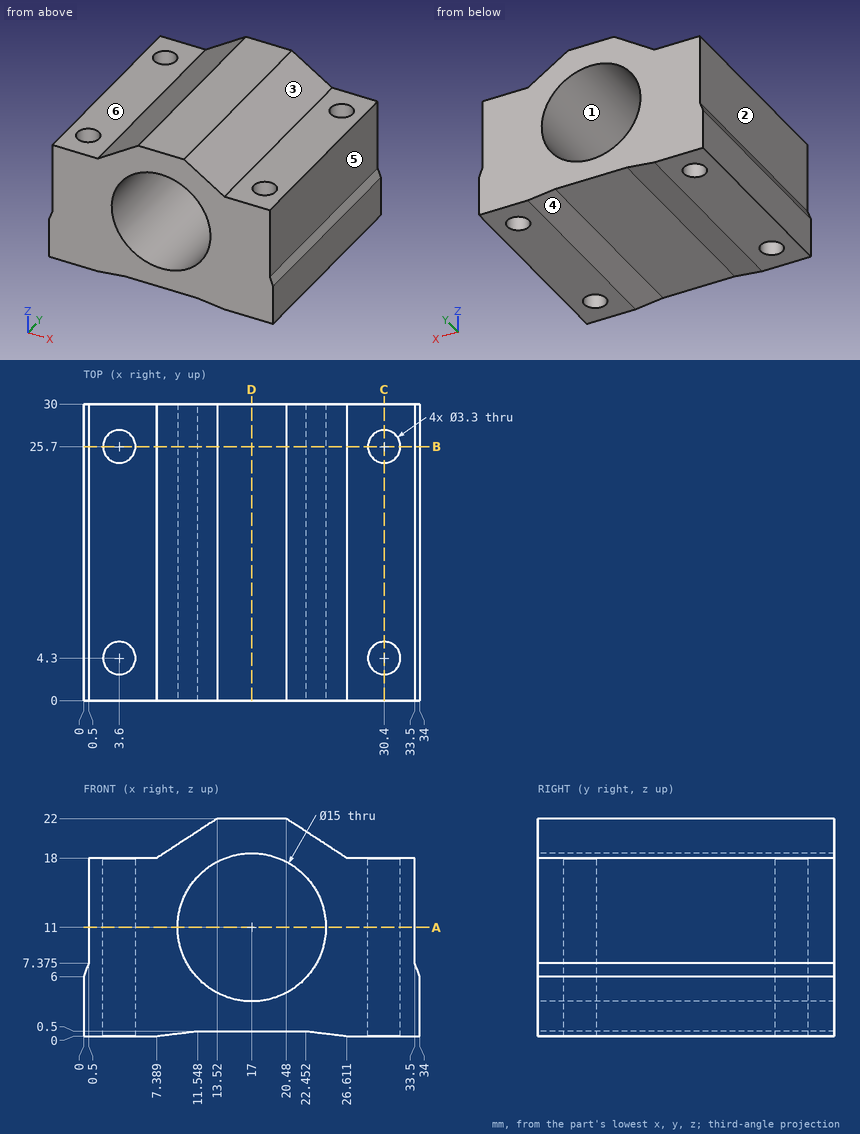
Study the drawing (mm; zero at the part's minimum x, y, z) and answer. A direction names the side the tool comes from. Coordinates: 2 decimals unless noted, no trailing zeros. Write each loop counter-clockwise with the first axis right and the second up, starting at its lowest first coordinate (ties: lowest second). Pieces come first, ordered by that corner, then holes. Notation, with made-up numbers: M 58.5,40.25 L 72.5,40.25 A23 ccw 72.5,59.25 Z; hole C 42.5,23 d1. An arc over 180 degrees is marked long. Write each question's results on one line, items separated by ' | '.
Item 1: Given P1, Ø8, axis at x = 8.5, y = 27, coming from the -Z side; P2, Ø2.5, axis at x = 3.6, y = 4.3, coming from the +Z side; P3, Ø5.5, axis at x = 19, y = 9.5, coming from the -Z side; P4, Ø8, axis at x = 7, y = 20, coming from the +Z side (1 decimal), each flat-ended and moving along its own axis, determine where each tip first touches the part or whether it passes through.
Answer below:
P1: z = 0 | P2: through | P3: z = 0.5 | P4: z = 20.4
Item 2: For a pull along X with two mould halves and no side action, classify the marked faces 1, 2 and 3 as released by +X, released by -X, zero draft, split by the parting line, or undercut.
Answer below:
face 1: undercut | face 2: released by -X | face 3: released by +X
Item 3: The part is cut by section D-D on x = 17. Determine the outline of the cut face in (y, z).
Answer below:
outline: M 0,0.5 L 30,0.5 L 30,3.5 L 0,3.5 Z; M 0,18.5 L 30,18.5 L 30,22 L 0,22 Z
Item 4: The part is cut by section A-A on z = 11. Determine the outline of the cut face in (x, y).
Answer below:
outline: M 0.5,0 L 9.5,0 L 9.5,30 L 0.5,30 Z; M 24.5,0 L 33.5,0 L 33.5,30 L 24.5,30 Z; hole C 3.6,4.3 d3.3; hole C 3.6,25.7 d3.3; hole C 30.4,4.3 d3.3; hole C 30.4,25.7 d3.3
Item 5: Which of the six approach directions +Z, -Z, +X, -X, +Y, -Y give full straight-line access (tool end or side, diameter ignored) to the marked faces 4, 5 and 6?
Answer below:
face 4: -Z, +Y, -Y | face 5: +Z, +X, +Y, -Y | face 6: +Z, -X, +Y, -Y
Item 6: The part is cut by section C-C on x = 30.4. Determine the outline of the cut face in (y, z), and give its area (3 significant figures).
Answer below:
outline: M 0,0 L 2.65,0 L 2.65,18 L 0,18 Z; M 5.95,0 L 24.05,0 L 24.05,18 L 5.95,18 Z; M 27.35,0 L 30,0 L 30,18 L 27.35,18 Z | area: 421 mm2
Item 7: Consider probe 1 along Y at (x, z) = (3.6, 4); probe 2 along Y at (x, z) = (3, 11.25); probe 3 along X at (y, z) = (25, 3.25) (1 decimal). Determine where each line is inside the solid, lowest interval first. Write a range as [from, to].
Answer below:
probe 1: [0, 2.65], [5.95, 24.05], [27.35, 30] | probe 2: [0, 2.76], [5.84, 24.16], [27.24, 30] | probe 3: [0, 2.1], [5.1, 28.9], [31.9, 34]
Item 8: The part is cut by section B-B on y = 25.7. State how many separate pieces and enclosed holes the cut face has, and give its area (3 significant figures).
Answer below:
separate pieces: 3 | enclosed holes: 1 | area: 350 mm2
